Design review of the part built by this model. Coordinates are the model's own, in mm. A direction names the side the tool comes from. Round coordinates to 2 decimals unless told otherwise and drop trailing zeros. Loops run counter-clockwise (first coordinate to the right, second up) from the corner with the lowest first, then second, coordinate; pieces in that order, holes last. Notation, with made-up numbers: (41, 60.25) - (65, 60.25) arc R21 cw to (65, 75.25) - close; hole circle Ø10 at (11.5, -1). An arc over 180 degrees is marked (long way). Return JSON: item names as keys, results as strings. Group by question number.
Autodesk Inventor part; units mm, degrees
ref_plane "YZ Plane" through (0, 0, 0) normal (1, 0, 0) x (0, 1, 0)
ref_plane "XZ Plane" through (0, 0, 0) normal (0, 1, 0) x (-1, 0, 0)
ref_plane "XY Plane" through (0, 0, 0) normal (0, 0, 1) x (1, 0, 0)
sketch "Sketch2" plane through (0, 0, 0) normal (0, 1, 0) x (-1, 0, 0)
  line L0 (0, 0) -> (-59, 0)
  line L1 (-59, 0) -> (-59, 73)
  line L2 (-59, 73) -> (0, 73)
  line L3 (0, 73) -> (0, 0)
  dimension "d0" = 59
  dimension "d1" = 73
extrude "Extrusion1" add sketch "Sketch2" along normal blind 18
shell "Shell1" thickness 3 removed faces 1 at (19.6667, 18, 24.3333)
sketch "Sketch4" plane through (59, 0, 0) normal (0, 0, -1) x (-1, 0, 0)
  point P0 (59, 0)
sketch "Sketch5" plane through (3, 3, 3) normal (0, 0, 1) x (1, 0, 0)
  line L0 (0, 0) -> (0, 15)
  line L1 (0, 15) -> (53, 15)
  line L2 (0, 0) -> (53, 0)
  line L3 (53, 0) -> (53, 15)
  line L4 (53, 15) -> (0, 15)
  line L5 (0, 15) -> (0, 0)
  point P0 (-3, -3)
extrude "Extrusion3" cut sketch "Sketch5" against normal blind 10
properties part number "arduino array box v02"
Q1. Add section B-B, the plane z = 47.5. State the section outline as (x, y) points.
Q2. For line 1 (X direction, y = 5, z = 57); line 2 (Z direction, x = 54, y = 16.75); line 3 (Y direction, x = 43.5, z = 6.5), list the stretches that pass through material, from the lowest coordinate up.
Q3. Insertion check: pin 1 Ø4.5 at (x, y) = (24, 9) entering from -Z; pin 2 Ø16 at (x, z) = (39, 40) entering from +Y. Each pin has a flat end and moves straight along its axis. Give the tip position at first contact, or say it passes through.
Q4. Draft analysis for pull direction X (two halves, no side actions). For faces 3 (the flat face through (59, 9, 36)), 4 (the flat face through (29, 3, 35)), 5 (the flat face through (30, 9, 73)), 6 (the flat face through (56, 10, 35)), state which applies: pulls with the +X half, pulls with the -X half, needs draft (parallel to the pull), parting line crosses it, or undercut.
Q5. Add section C-C, the plane x = 49.5. State the section outline as (y, z) points.
Q6. Add section A-A, the plane y = 14.25. State the section outline as (x, z) points.
Q7. Tool access review of faces 1 (the flat face through (3, 10, 35)), 2 (the flat face through (29, 2, 0)): name each direction out of +Z, -Z, +X, -X, +Y, -Y from which nothing blocks a thin tool from reaching the whole face with its end or side.
Evaluation:
{
 "1": {"outline": "(0, 0) - (59, 0) - (59, 18) - (56, 18) - (56, 3) - (3, 3) - (3, 18) - (0, 18) - close"},
 "2": {"line 1": "0 to 3, 56 to 59", "line 2": "70 to 73", "line 3": "0 to 3"},
 "3": {"pin 1": "z = 70", "pin 2": "y = 3"},
 "4": {"face 3": "pulls with the +X half", "face 4": "undercut", "face 5": "needs draft", "face 6": "undercut"},
 "5": {"outline": "(0, 0) - (3, 0) - (3, 70) - (18, 70) - (18, 73) - (0, 73) - close"},
 "6": {"outline": "(0, 0) - (3, 0) - (3, 70) - (56, 70) - (56, 0) - (59, 0) - (59, 73) - (0, 73) - close"},
 "7": {"face 1": "-Z, +Y", "face 2": "-Z, +X, -X, +Y, -Y"}
}
